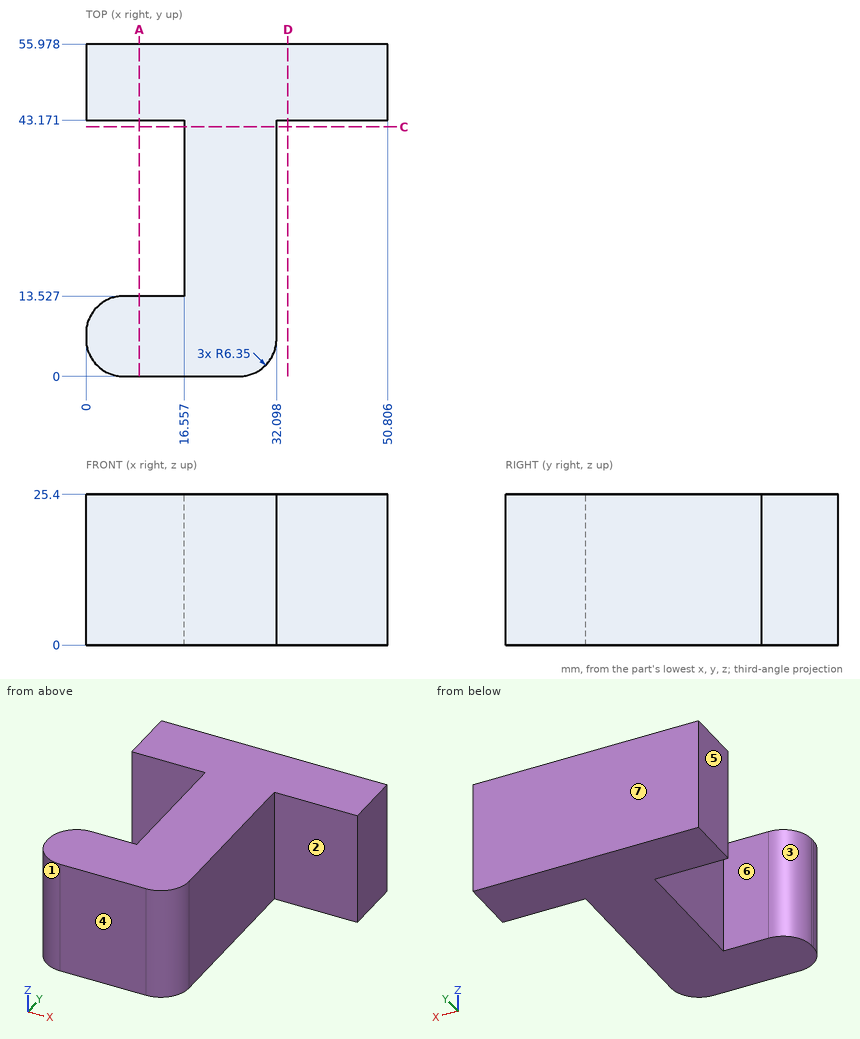
Input: dimensioned drawing with shaded views. Units: mm. Origin: part minimum x, y, z. A direction names the side the tool comes from. Round coordinates to 2 decimals unless told otherwise and drop trailing zeros. Write each loop counter-clockwise with the first axis right and the second up, starting at its lowest first coordinate (ties: lowest second). Pieces come first, ordered by that corner, then holes. Notation, with made-up numbers: (-16.75, -37.75) - (0.25, -37.75) arc R20 ccw to (0.25, -9.75) - close; hole circle Ø4 at (15.25, 15.5). An arc over 180 degrees is marked (long way). Write item = value, one per line.
(1) Section query A-A on x = 9. Output: boundary loops of the cut face in (y, z).
Geometry check:
outline = (0, 0) - (13.53, 0) - (13.53, 25.4) - (0, 25.4) - close; (43.17, 0) - (55.98, 0) - (55.98, 25.4) - (43.17, 25.4) - close
(2) Section query C-C on y = 42. Output: boundary loops of the cut face in (x, z).
Geometry check:
outline = (16.56, 0) - (32.1, 0) - (32.1, 25.4) - (16.56, 25.4) - close
(3) Contact query for flat-ended pins moving along their axis: pin 1 Ø12.5 at (y, z) = (23, 11.5) entering from +X; pin 2 Ø1 at (y, z) = (8, 13) entering from -X; pin 3 Ø7.5 at (y, z) = (24.5, 11.5) entering from -X. Output: stop coordinate, or through.
Geometry check:
pin_1 = 32.1
pin_2 = 0.01
pin_3 = 16.56
(4) Pull-direction query (Y, two-part tool) for the marked faces 4, 5, 6 and 7; classes: +Y half, -Y half, draft (parallel to the pull), parting line (faces both ways), or undercut.
Geometry check:
face_4 = -Y half
face_5 = draft
face_6 = undercut
face_7 = +Y half
(5) Access query for the marked faces 1, 2 and 3. Directions: +Z, -Z, +X, -X, +Y, -Y. A direction counts if a zero-diameter tool reaches every point of the face in a straight line with its end or side. Return the directions, or none.
Geometry check:
face_1 = +Z, -Z, -X, -Y
face_2 = +Z, -Z, +X, -Y
face_3 = +Z, -Z, -X
(6) Section query D-D on x = 34. Output: boundary loops of the cut face in (y, z).
Geometry check:
outline = (43.17, 0) - (55.98, 0) - (55.98, 25.4) - (43.17, 25.4) - close
(7) Material intervals for probe 1 along Y at (x, z) = (10.5, 2.75); probe 2 along X at (y, z) = (33.5, 14.5); probe 3 along Y at (x, z) = (3, 5) (1 decimal), sorted ascending.
Geometry check:
probe_1 = 0 to 13.53, 43.17 to 55.98
probe_2 = 16.56 to 32.1
probe_3 = 1 to 12.6, 43.2 to 56
